Study the drawing (mm; zero at the part's minimum x, y, z) and answer. A direction names the side the tool comes from. Round coordinates to 2 decimals unless told otherwise and drop trailing zeros. Write each loop counter-clockwise with the first axis right and the second up, starting at its lowest first coordinate (ties: lowest second). Pieces come first, ordered by that corner, then holes. Notation, with made-up numbers: (76, 19.25) -> (105, 19.25) arc R16 cw to (105, 38.25) -> close; hole circle Ø10 at (-38, 87.5). An arc over 180 degrees is marked (long way). Write each question's results on one line, items separated by ' | '. Start each with the question number.
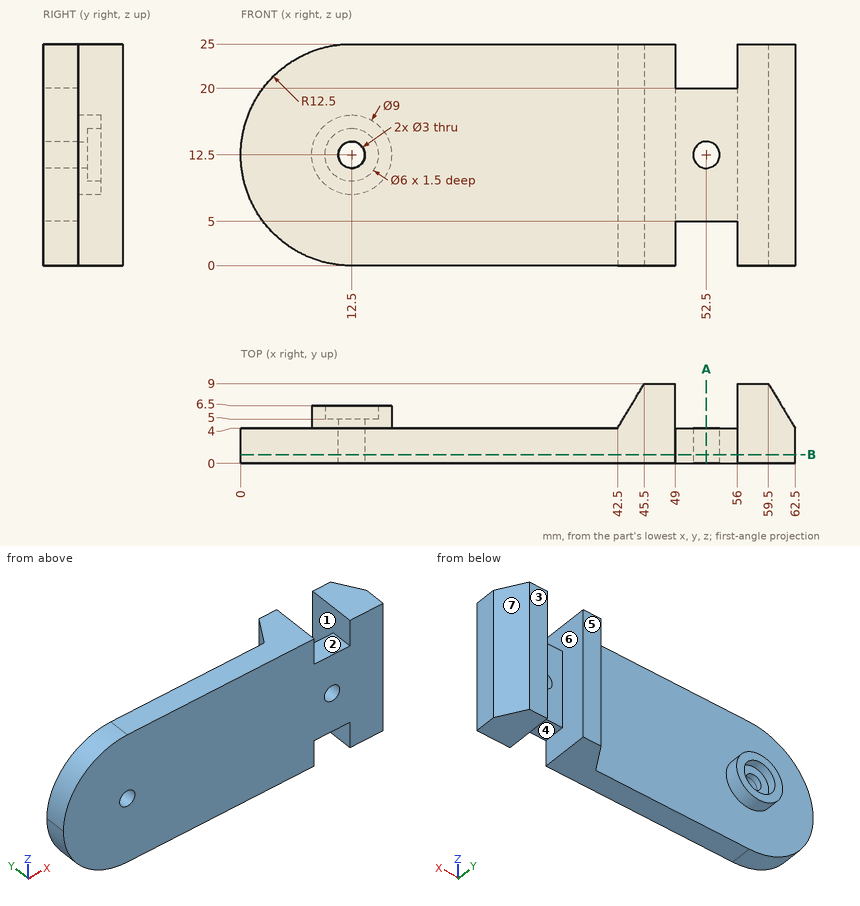
Q1. Each of these flat-tipped pins is pushed along its axis until it touches: pin 1 (5 mm diameter, centred on x = 11, z = 13.5, fed in from +Y); pin 2 (2 mm diameter, centred on y = 6.5, z = 19, fed in from -X); pin 3 (1.2 mm diameter, centred on x = 51.5, y = 1.5, fed in from -Z). Where does it stop, or does it pass through?
Q2. Determine the mould class of the marked faces 5, 6 and 7 for opening direction X: pulls with the +X half, pulls with the -X half, needs draft (parallel to the pull), parting line crosses it, or undercut.
Q3. The part is cut by section A-A, the plane x = 52.5. Write down the section's boundary in (y, z).
Q4. The part is cut by section B-B, the plane y = 1. Write down the section's boundary in (x, z).
Q5. For the marked faces 1, 2, 3 and 4, determine the directions among +Z, -Z, +X, -X, +Y, -Y from which every point of the face is accessible in a straight line to the end or side of a thin tool.
Q6. Find the intervals of material crossed by line 1 (Z direction, x = 52.5, y = 1.85); line 2 (X direction, y = 4.55, z = 12.5); line 3 (X direction, y = 4.75, z = 13), in increasing order.
Answers follow:
1) pin 1: y = 6.5 | pin 2: x = 43.4 | pin 3: z = 5
2) face 5: needs draft | face 6: undercut | face 7: pulls with the +X half
3) outline: (0, 5) -> (4, 5) -> (4, 11) -> (0, 11) -> close; (0, 14) -> (4, 14) -> (4, 20) -> (0, 20) -> close
4) outline: (12.5, 0) -> (49, 0) -> (49, 5) -> (56, 5) -> (56, 0) -> (62.5, 0) -> (62.5, 25) -> (56, 25) -> (56, 20) -> (49, 20) -> (49, 25) -> (12.5, 25) arc R12.5 ccw to start; hole circle Ø3 at (12.5, 12.5); hole circle Ø3 at (52.5, 12.5)
5) face 1: +Y | face 2: +Z, +Y, -Y | face 3: +Z, -Z, +X, -X, +Y | face 4: -Z, +Y, -Y
6) line 1: 5 to 11, 14 to 20 | line 2: 8 to 11, 14 to 17, 42.83 to 49, 56 to 62.17 | line 3: 8.03 to 11.09, 13.91 to 16.97, 42.95 to 49, 56 to 62.05
